Autodesk Inventor part; units mm, degrees
ref_plane "ZS1_XY" through (0, 0, 0) normal (1, 0, 0) x (0, 0, -1)
ref_plane "ZS1_YZ" through (0, 0, 0) normal (0, 0, -1) x (0, 1, 0)
ref_plane "ZS1_ZX" through (0, 0, 0) normal (0, 1, 0) x (1, 0, 0)
sketch "Skizze_1" plane through (0, 0, 0) normal (1, 0, 0) x (0, 1, 0)
  arc A0 (3, 6.4) -> (-3, 6.4) centre (0, 6.4) ccw
  line L0 (-3, 6.4) -> (-3, 0)
  arc A1 (-3, 0) -> (3, 0) centre (0, 0) ccw
  line L1 (3, 0) -> (3, 6.4)
extrude "Extrusion1" add sketch "Skizze_1" along normal mid plane 3
sketch "Skizze_2" plane through (0, 0, 0) normal (0, 1, 0) x (-1, 0, 0)
  line L0 (-10, 0) -> (10, 0)
  line L1 (10, 0) -> (10, -1.215)
  line L2 (10, -1.215) -> (-10, -1.215)
  line L3 (-10, -1.215) -> (-10, 0)
  line L4 (-10, 0) -> (10, 0)
revolve "Revolution1" cut sketch "Skizze_2" angle 360 about axis through (10, 0, 0) along (1, 0, 0)
sketch "Skizze_3" plane through (0, 0, 0) normal (0, 1, 0) x (-1, 0, 0)
  line L0 (-10, 6.4) -> (10, 6.4)
  line L1 (10, 6.4) -> (10, 5.185)
  line L2 (10, 5.185) -> (-10, 5.185)
  line L3 (-10, 5.185) -> (-10, 6.4)
  line L4 (-10, 6.4) -> (10, 6.4)
revolve "Revolution2" cut sketch "Skizze_3" angle 360 about axis through (10, 0, 6.4) along (1, 0, 0)
ref_plane "ZS1_XY" through (0, 0, 0) normal (1, 0, 0) x (0, 0, -1)
ref_plane "ZS1_YZ" through (0, 0, 0) normal (0, 0, -1) x (0, 1, 0)
ref_plane "ZS1_ZX" through (0, 0, 0) normal (0, 1, 0) x (1, 0, 0)
ref_plane "ZS2_XY" through (0, 0, 6.4) normal (1, 0, 0) x (0, 0, -1)
ref_plane "ZS2_YZ" through (0, 0, 6.4) normal (0, 0, -1) x (0, 1, 0)
ref_plane "ZS2_ZX" through (0, 0, 6.4) normal (0, 1, 0) x (1, 0, 0)
properties part number "205-S-ZS"
Input: part model. Units: mm. Frame: model coordinates. Give positions to 0.01 mm unless a question says otherwise; leave off trailing zeros. Order: outer loops, then holes, each group sorted by start corner. A loop starts at its lowest first (then second) coordinate and runs counter-clockwise, first axis right, second up.
1. Cut plane A-A (y = 0). Return loops of the section in (x, z) (3 decimals), and give its area (3 significant figures).
Computed:
outline: (-1.5, -3) - (1.5, -3) - (1.5, -1.215) - (-1.5, -1.215) - close; (-1.5, 1.215) - (1.5, 1.215) - (1.5, 5.185) - (-1.5, 5.185) - close; (-1.5, 7.615) - (1.5, 7.615) - (1.5, 9.4) - (-1.5, 9.4) - close
area: 22.6 mm2
2. Cut plane B-B (z = 7.25). Return loops of the section in (x, y).
Computed:
outline: (-1.5, -2.88) - (1.5, -2.88) - (1.5, -0.87) - (-1.5, -0.87) - close; (-1.5, 0.87) - (1.5, 0.87) - (1.5, 2.88) - (-1.5, 2.88) - close
3. Draft query along Y for faces 1 (the face through (0.021, 0.053, 7.614)), 2 (the face through (0, 0, -3)), 3 (the face through (-1.5, 0, 3)). Return one class per face: released by +Y, released by -Y, zero draft, split by the parting line, or undercut.
Computed:
face 1: undercut
face 2: split by the parting line
face 3: zero draft
4. Pin query (flat end, axial travel): pin 1 Ø3 at (y, z) = (0, 0) entering from -X; pin 2 Ø1.5 at (x, y) = (0.5, 1) entering from -Z. Return the tip coordinate at first contact, or that it passes through.
Computed:
pin 1: stops at x = -1.5
pin 2: stops at z = -2.99
5. Cut plane D-D (z = -1). Return loops of the section in (x, y), and give its area (3 significant figures).
Computed:
outline: (-1.5, -2.83) - (1.5, -2.83) - (1.5, -0.69) - (-1.5, -0.69) - close; (-1.5, 0.69) - (1.5, 0.69) - (1.5, 2.83) - (-1.5, 2.83) - close
area: 12.8 mm2
6. Cut plane C-C (x = -1.25). Return loops of the section in (y, z) (3 decimals), and give its area (3 significant figures).
Computed:
outline: (-3, 0) arc R3 ccw to (3, 0) - (3, 6.4) arc R3 ccw to (-3, 6.4) - close; hole circle Ø2.43 at (0, 0); hole circle Ø2.43 at (0, 6.4)
area: 57.4 mm2
7. Line query: probe 1 along Y at (x, z) = (0.4, 6.4) (3 decimals); probe 2 along Z at (x, y) = (-0.6, 0.55); probe 3 along Z at (x, y) = (0.4, 0.95). Output: solid intervals per line, ascending.
Computed:
probe 1: y = -3 to -1.215, 1.215 to 3
probe 2: z = -2.95 to -1.08, 1.08 to 5.32, 7.48 to 9.35
probe 3: z = -2.85 to -0.76, 0.76 to 5.64, 7.16 to 9.25
